Check sheet for the modelled part. Datum: model origin and axes. Units: mm. A direction names the side the tool comes from. Give positions to 0.01 mm unless a question says otherwise; leave off trailing zeros. Loops run counter-clockwise (first coordinate to the right, second up) from the corner with the lowest first, then second, coordinate; pieces in that order, holes last. Notation, with made-up numbers: (-6, 89) -> (29, 89) arc R15 cw to (29, 115) -> close; hole circle Ø5 at (71.5, -30). An arc over 180 degrees is marked (long way). Write each question's results on one line, items separated by ' | '. Start each with the question number.
1. Gauge pin test, flat ends, axial feed: pin 1 Ø3 at (x, z) = (52.5, 9.5) entering from -Y; pin 2 Ø3 at (x, y) = (1, 0) entering from -Z; pin 3 Ø3 at (x, y) = (47.5, -107.5) entering from +Z. Record the tip position at first contact, or that the pin passes through.
2. Material ranges on L1, parallel to X at y = -69, z = 4 (3 decimals); L2, parallel to Y at x = 18, z = 12; L3, parallel to Y at x = 43, z = 8.25, recorded low to high. Write a range as from..to.
3. Cross-section at B-B on x = 12.5. Record the boundary of the cut face in (y, z), and give its area (3 significant figures).
4. Tool access check on faces 1 (the face through (-0.65, -104.702, 1.528)), 2 (the face through (38.742, -108, 9)), 3 (the face through (47, -112.631, 5)), 4 (the face through (91.225, -55, 8)). Record the directions out of +Z, -Z, +X, -X, +Y, -Y that give a thin tool (end or side, any length) a straight path to the whole face; none if there is none.
5. Cross-section at C-C on z = 11.25. Record the boundary of the cut face in (x, y) (3 decimals), and give its area (3 significant figures).
6. Mould release check, pull along X, two halves, no side actions. Record for faces 5 (the face through (48, -108, 5.5)), 6 (the face through (47, -53, 0)), 7 (the face through (-3, 4, 6)): +X half, -X half, draft (parallel to the pull), parting line (faces both ways), or undercut.
7. Cross-section at A-A on y = -99. Record the boundary of the cut face in (x, z) (3 decimals).
from build123d import *

# Parameters (mm, degrees)
SKETCH_R        = 1.7
PAD_DEPTH       = 13
SKETCH001_W     = 86.725
SKETCH001_H     = 98.631
POCKET_DEPTH    = 10
SKETCH002_W     = 18.5
SKETCH002_H     = 7.5
POCKET001_DEPTH = 11
SKETCH003_R     = 3
POCKET002_DEPTH = 3.1


with BuildPart() as part:
    # Sketch → Pad (new body)
    with BuildSketch(Plane.XY):
        with BuildLine():
            Line((-5, 0), (-5, -107.631))
            ThreePointArc((-5, -107.631), (-3.535534, -111.166534), (0, -112.631))
            Line((0, -112.631), (95.725, -112.631))
            ThreePointArc((95.725, -112.631), (99.260534, -111.166534), (100.725, -107.631))
            Line((100.725, -107.631), (100.725, 0))
            ThreePointArc((100.725, 0), (99.260534, 3.535534), (95.725, 5))
            Line((95.725, 5), (0, 5))
            ThreePointArc((0, 5), (-3.535534, 3.535534), (-5, 0))
        make_face()
        Circle(SKETCH_R, mode=Mode.SUBTRACT)
        with Locations((95.725, 0)):
            Circle(SKETCH_R, mode=Mode.SUBTRACT)
        with Locations((95.725, -107.631)):
            Circle(SKETCH_R, mode=Mode.SUBTRACT)
        with Locations((0, -107.631)):
            Circle(SKETCH_R, mode=Mode.SUBTRACT)
    extrude(amount=PAD_DEPTH)

    # Sketch001 (on Face14 of Pad) → Pocket (cut)
    with BuildSketch(Plane.XY.offset(13)):
        with Locations((47.8625, -53.8155)):
            Rectangle(SKETCH001_W, SKETCH001_H)
    extrude(amount=-POCKET_DEPTH, mode=Mode.SUBTRACT)

    # Sketch002 (on Face7 of Pocket) → Pocket001 (cut)
    with BuildSketch(Plane.XZ.offset(112.631)):
        with Locations((47.992, 9.25)):
            Rectangle(SKETCH002_W, SKETCH002_H)
    extrude(amount=-POCKET001_DEPTH, mode=Mode.SUBTRACT)

    # Sketch003 (on Face4 of Pocket001) → Pocket002 (cut)
    with BuildSketch(Plane(origin=(0, 0, 0), x_dir=(1, 0, 0), z_dir=(0, 0, -1))):
        with Locations((0, 107.631)):
            Circle(SKETCH003_R)
        with Locations((95.725, 107.631)):
            Circle(SKETCH003_R)
        with Locations((95.725, 0)):
            Circle(SKETCH003_R)
        Circle(SKETCH003_R)
    extrude(amount=-POCKET002_DEPTH, mode=Mode.SUBTRACT)


solid = part.part
Geometry says:
1) pin 1: y = -4.5 | pin 2: z = 3.1 | pin 3: z = 5.5
2) L1: -5..4.5, 91.225..100.725 | L2: -112.63..-103.13, -4.5..5 | L3: -4.5..5
3) outline: (-112.63, 0) -> (5, 0) -> (5, 13) -> (-4.5, 13) -> (-4.5, 3) -> (-103.13, 3) -> (-103.13, 13) -> (-112.63, 13) -> close | area: 543 mm^2
4) face 1: -Z | face 2: +Z, -Y | face 3: +Z, -Z, +X, -X, -Y | face 4: +Z
5) outline: (-5, -107.631) arc R5 ccw to (0, -112.631) -> (38.742, -112.631) -> (38.742, -103.131) -> (4.5, -103.131) -> (4.5, -4.5) -> (91.225, -4.5) -> (91.225, -103.131) -> (57.242, -103.131) -> (57.242, -112.631) -> (95.725, -112.631) arc R5 ccw to (100.725, -107.631) -> (100.725, 0) arc R5 ccw to (95.725, 5) -> (0, 5) arc R5 ccw to (-5, 0) -> close; hole circle Ø3.4 at (0, -107.631); hole circle Ø3.4 at (0, 0); hole circle Ø3.4 at (95.725, -107.631); hole circle Ø3.4 at (95.725, 0) | area: 3,650 mm^2
6) face 5: undercut | face 6: draft | face 7: -X half
7) outline: (-5, 0) -> (100.725, 0) -> (100.725, 13) -> (91.225, 13) -> (91.225, 3) -> (4.5, 3) -> (4.5, 13) -> (-5, 13) -> close
